Check sheet for the modelled part. Datum: model origin and axes. Units: mm. Round coordinates to 2 decimals unless told otherwise and drop trailing zeros. Write each loop counter-clockwise with the first axis right and the second up, starting at its lowest first coordinate (ties: lowest second). Pieces come first, ordered by that corner, then holes. Notation, with made-up numbers: M -17,51 L 11,51 A22 cw 11,73 Z; hole C -27,74 d11. An arc over 180 degrees is marked long. Answer in a Markdown table with one row per item.
```python
from build123d import *

# Parameters (mm, degrees)
SKETCH1_W                 = 42
SKETCH1_H                 = 42
BOSS_EXTRUDE1_DEPTH       = 4
SKETCH2_R                 = 3
CUT_EXTRUDE1_DEPTH        = 16
F_5_0MM_DOWEL_HOLE1_D     = 5
F_5_0MM_DOWEL_HOLE1_DEPTH = 25
F_5_0MM_DOWEL_HOLE1_TIP   = 1.502151548


with BuildPart() as part:
    # Sketch1 → Boss-Extrude1 (new body)
    with BuildSketch(Plane(origin=(0, 0, 0), x_dir=(1, 0, 0), z_dir=(0, 1, 0))):
        with Locations((1.276868931, -0.638434466)):
            Rectangle(SKETCH1_W, SKETCH1_H)
    extrude(amount=BOSS_EXTRUDE1_DEPTH)

    # Sketch2 → Cut-Extrude1 (cut)
    with BuildSketch(Plane(origin=(0, 4, 0), x_dir=(1, 0, 0), z_dir=(0, 1, 0))):
        with Locations(Location((1.276868931, -0.638434466, 0), (0, 0, 270))):
            Circle(SKETCH2_R)
    extrude(amount=-CUT_EXTRUDE1_DEPTH, mode=Mode.SUBTRACT)

    # Ø5.0mm Dowel Hole1
    with Locations(Plane(origin=(0, 4, 0), x_dir=(1, 0, 0), z_dir=(0, 1, 0))):
        with Locations((-15.111953931, -10.525403014), (-15.111953931, 9.248534083), (17.665691793, 9.248534083), (17.665691793, -10.525403014)):
            Hole(F_5_0MM_DOWEL_HOLE1_D / 2, depth=F_5_0MM_DOWEL_HOLE1_DEPTH)
            with Locations((0, 0, -(F_5_0MM_DOWEL_HOLE1_DEPTH + F_5_0MM_DOWEL_HOLE1_TIP / 2))):  # 118° drill point
                Cone(0, F_5_0MM_DOWEL_HOLE1_D / 2, F_5_0MM_DOWEL_HOLE1_TIP, mode=Mode.SUBTRACT)


solid = part.part
```
1. Section check C-C, the plane x = -14. Record the cut outline in (y, z), and give its area (3 significant figures).
Found:
| item | result |
|---|---|
| outline | M 0,-20.36 L 4,-20.36 L 4,-11.49 L 0,-11.49 Z; M 0,-7.01 L 4,-7.01 L 4,8.29 L 0,8.29 Z; M 0,12.76 L 4,12.76 L 4,21.64 L 0,21.64 Z |
| area | 132 mm2 |
2. Section check A-A, the plane z = 9. Record the cut outline in (x, y) (3 decimals).
Found:
| item | result |
|---|---|
| outline | M -19.723,0 L -17.093,0 L -17.093,4 L -19.723,4 Z; M -13.131,0 L 15.685,0 L 15.685,4 L -13.131,4 Z; M 19.646,0 L 22.277,0 L 22.277,4 L 19.646,4 Z |
3. Section check B-B, the plane x = 3.5. Record the cut outline in (y, z).
Found:
| item | result |
|---|---|
| outline | M 0,-20.36 L 4,-20.36 L 4,-1.38 L 0,-1.38 Z; M 0,2.65 L 4,2.65 L 4,21.64 L 0,21.64 Z |
4. Draft check along Z on faces 1 (the face through (-13.269, 1.972, 8.836)), 2 (the face through (22.277, 2, 1)), 3 (the face through (1, 2, 21.638)), 4 (the face through (16.51, 1.97, -7.03)). Enter one of: +Z half, -Z half, draft (parallel to the pull), parting line (faces both ways), or undercut.
Found:
| item | result |
|---|---|
| face 1 | undercut |
| face 2 | draft |
| face 3 | +Z half |
| face 4 | undercut |
5. Scan lines: L1, parallel to Z at x = 1.5, y = 0.5; L2, parallel to X at y = 3.35, z = -10; L3, parallel to X at y = 2.65, z = -8. Record each from-to range of solid material in increasing order.
Found:
| item | result |
|---|---|
| L1 | z = -20.36 to -2.35, 3.63 to 21.64 |
| L2 | x = -19.72 to -17.5, -12.73 to 15.28, 20.05 to 22.28 |
| L3 | x = -19.72 to -17.28, -12.95 to 15.5, 19.83 to 22.28 |
6. Section check D-D, the plane z = 1. Record the cut outline in (x, y) (3 decimals).
Found:
| item | result |
|---|---|
| outline | M -19.723,0 L -1.701,0 L -1.701,4 L -19.723,4 Z; M 4.255,0 L 22.277,0 L 22.277,4 L 4.255,4 Z |
